Answer from the drawing. Dimensions are ordinates in mm from the lowest x, y and z of the part. A direction names the side the tool comes from. Give positions to 0.01 mm unless a question says otherwise; leave off trailing zeros. Loops run counter-clockwise (first coordinate to the right, second up) from the corner with the lowest first, then second, coordinate; pieces in that order, holes last. Notation, with made-up numbers: (40, 5.25) - (69, 5.25) arc R22 ccw to (69, 27.25) - close; hole circle Ø3 at (-7.5, -21). An arc over 180 degrees is marked (long way). One line per item, written item: value.
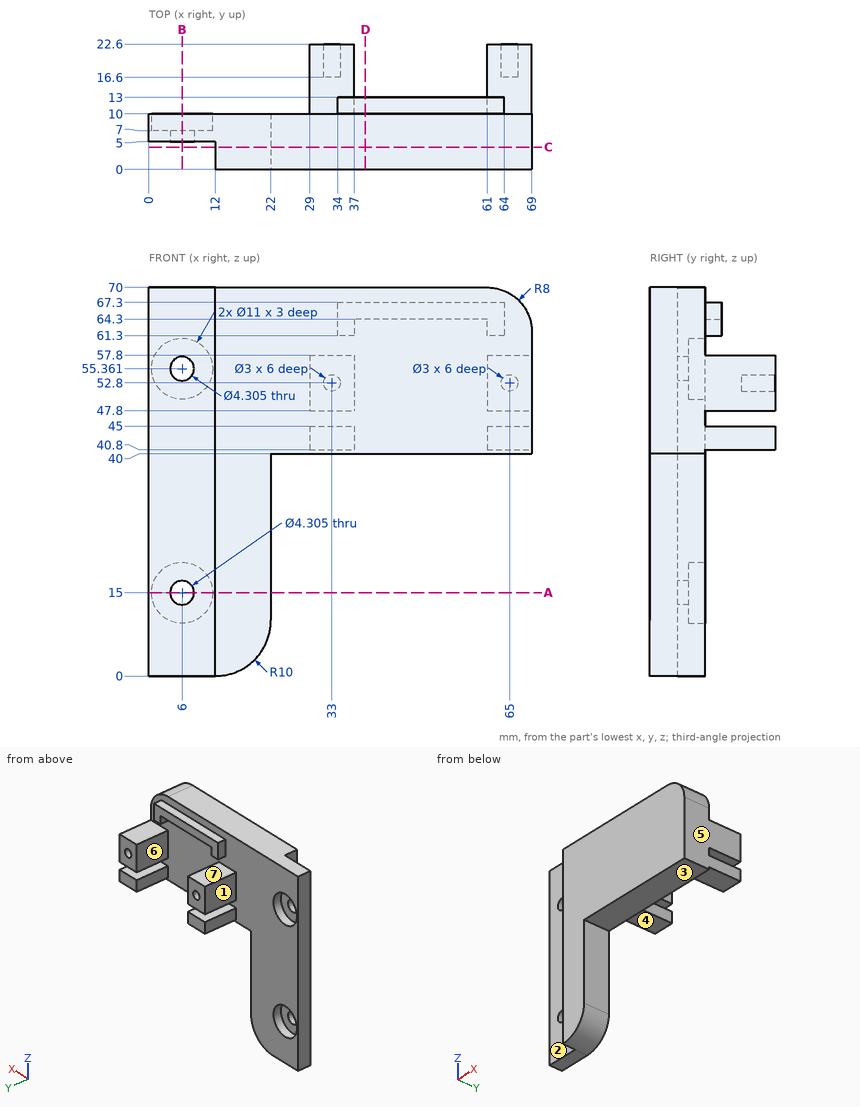
1. For the marked faces 1, 2, 3 and 4, determine the directions among +Z, -Z, +X, -X, +Y, -Y from which every point of the face is accessible in a straight line to the end or side of a thin tool.
Output:
face 1: +Z, -Z, -X, +Y
face 2: +Z, -Z, -X, -Y
face 3: -Z, +X, +Y, -Y
face 4: -Z, +X, -X, +Y
2. Section A-A (z = 15) is taken. Write down the section's boundary in (x, y), and give its area (3 significant figures).
Output:
outline: (0, 5) - (3.85, 5) - (3.85, 7) - (0.5, 7) - (0.5, 10) - (0, 10) - close; (8.15, 5) - (12, 5) - (12, 0) - (22, 0) - (22, 10) - (11.5, 10) - (11.5, 7) - (8.15, 7) - close
area: 118 mm²
3. Find the intervals of material crossed by line 1 along X through (y, z) = (20.7, 52.8); line 2 along Z through (x, y) = (6, 9.45); line 3 along Z through (x, y) = (33, 19.85), in increasing order.
Output:
line 1: x = 29 to 31.5, 34.5 to 37, 61 to 63.5, 66.5 to 69
line 2: z = 0 to 9.5, 20.5 to 49.86, 60.86 to 70
line 3: z = 40.8 to 45, 47.8 to 51.3, 54.3 to 57.8
4. The mould has two halves that part along X. Classify the marked faces 5, 6 and 7: released by +X, released by -X, zero draft, split by the parting line, or undercut.
Output:
face 5: released by +X
face 6: undercut
face 7: zero draft
5. Section C-C (y = 4) is taken. Write down the section's boundary in (x, z).
Output:
outline: (12, 0) arc R10 ccw to (22, 10) - (22, 40) - (69, 40) - (69, 62) arc R8 ccw to (61, 70) - (12, 70) - close
6. Section D-D (x = 39) is taken. Write down the section's boundary in (y, z).
Output:
outline: (0, 40) - (10, 40) - (10, 64.3) - (13, 64.3) - (13, 67.3) - (10, 67.3) - (10, 70) - (0, 70) - close
7. Flat-ended cylindrical pins translate along their axes: pin 1 Ø14.5 at (x, z) = (6, 15) entering from +Y; pin 2 Ø4 at (x, z) = (6, 15) entering from +Y; pin 3 Ø3 at (y, z) = (18.5, 51.5) entering from -X; pin 4 Ø2.5 at (x, z) = (65, 52.8) entering from +Y. Find the tip coordinate at first contact, or state that the pin passes through.
Output:
pin 1: stops at y = 10
pin 2: passes through
pin 3: stops at x = 29
pin 4: stops at y = 16.6
8. Section B-B (x = 6) is taken. Write down the section's boundary in (y, z).
Output:
outline: (5, 0) - (10, 0) - (10, 9.5) - (7, 9.5) - (7, 12.85) - (5, 12.85) - close; (5, 17.15) - (7, 17.15) - (7, 20.5) - (10, 20.5) - (10, 49.86) - (7, 49.86) - (7, 53.21) - (5, 53.21) - close; (5, 57.51) - (7, 57.51) - (7, 60.86) - (10, 60.86) - (10, 70) - (5, 70) - close
